Here's how the part is built. I have some questions about the finished solid (model axes, mm). Give positions to 0.01 mm unless a question says otherwise; leave off trailing zeros. Order: outer loops, then holes, each group sorted by start corner. A loop starts at its lowest first (then second) coordinate and runs counter-clockwise, first axis right, second up.
from build123d import *

# Parameters (mm, degrees)
MODEL_R             = 1.587496825
BOSS_EXTRUDE1_DEPTH = 2


with BuildPart() as part:
    # Model → Boss-Extrude1 (new body)
    with BuildSketch(Plane.XY):
        with BuildLine():
            Line((-146.653910016, 921.021419751), (-146.653491939, 987.021287754))
            Line((-146.653491939, 987.021287754), (-147.399894202, 987.021287754))
            ThreePointArc((-147.399894202, 987.021287754), (-150.935437408, 988.485719341), (-152.399999963, 992.021208297))
            ThreePointArc((-152.399999963, 992.021208297), (-153.278698205, 994.142573511), (-155.400063419, 995.021271753))
            Line((-155.400063419, 995.021271753), (-209.399816512, 995.021271753))
            ThreePointArc((-209.399816512, 995.021271753), (-211.521116241, 994.142638994), (-212.399879965, 992.021393514))
            ThreePointArc((-212.399879965, 992.021393514), (-213.864303366, 988.485858493), (-217.399777355, 987.021287754))
            ThreePointArc((-217.399777355, 987.021287754), (-220.228264308, 985.849690097), (-221.399861964, 983.021203145))
            Line((-221.399861964, 983.021203145), (-221.399861964, 925.021411752))
            ThreePointArc((-221.399861964, 925.021411752), (-220.228216634, 922.192969733), (-217.39973512, 921.02141975))
            ThreePointArc((-217.39973512, 921.02141975), (-213.864288435, 919.55683408), (-212.399879966, 916.021313993))
            ThreePointArc((-212.399879966, 916.021313993), (-211.521116244, 913.900068513), (-209.399816515, 913.021435753))
            Line((-209.399816515, 913.021435753), (-155.506885764, 913.021435753))
            ThreePointArc((-155.506885764, 913.021435753), (-155.475395221, 913.097173017), (-155.399490011, 913.128256561))
            ThreePointArc((-155.399490011, 913.128256561), (-155.324999759, 913.097438787), (-155.293258, 913.023337548))
            ThreePointArc((-155.293258, 913.023337548), (-153.267730715, 913.91115848), (-152.400955638, 915.945780743))
            ThreePointArc((-152.400955638, 915.945780743), (-152.427675956, 915.951027262), (-152.450799863, 915.965407327))
            ThreePointArc((-152.450799863, 915.965407327), (-152.470357006, 916.048810735), (-152.399429358, 916.096851124))
            ThreePointArc((-152.399429358, 916.096851124), (-150.946546283, 919.545844687), (-147.506710495, 921.020278673))
            ThreePointArc((-147.506710495, 921.020278673), (-147.476166718, 921.096209628), (-147.400849891, 921.128237863))
            ThreePointArc((-147.400849891, 921.128237863), (-147.324698014, 921.09729172), (-147.293071814, 921.021419751))
            Line((-147.293071814, 921.021419751), (-146.653910016, 921.021419751))
        make_face()
        with Locations((-208.399887964, 918.965401326)):
            Circle(MODEL_R, mode=Mode.SUBTRACT)
        with Locations((-157.399989964, 918.965401326)):
            Circle(MODEL_R, mode=Mode.SUBTRACT)
        with Locations((-208.399887964, 988.965261326)):
            Circle(MODEL_R, mode=Mode.SUBTRACT)
        with Locations((-157.399989964, 988.965261326)):
            Circle(MODEL_R, mode=Mode.SUBTRACT)
    extrude(amount=BOSS_EXTRUDE1_DEPTH)


solid = part.part
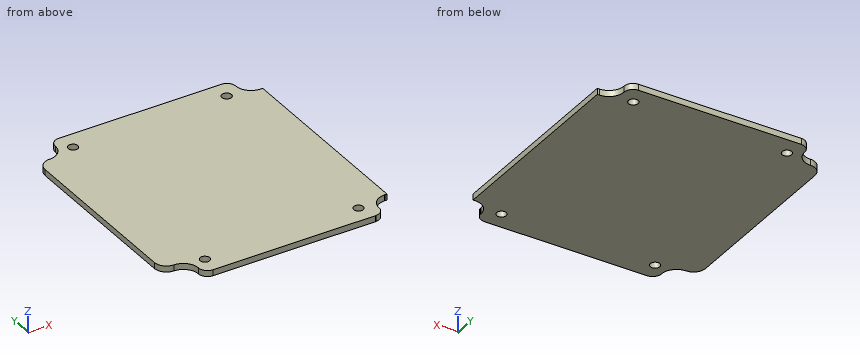
Q1. I'm going to push a flat-ended pin straight in: P1, Ø0.8, axis at x = -147, z = 1, coming from the +Y side. Where does the tip first touch, or does it pass through?
Filled sheet:
P1: stops at y = 987.02
Q2. If we section it at A-A on z = 0.3: Give the number of separate pieces and of enclosed holes in the cut face, plus the area to 3 significant figures.
Filled sheet:
separate pieces: 1
enclosed holes: 4
area: 5,870 mm2
Q3. I need wall thicknesses on L1, parallel to Y at x = -208, z = 1.25; L2, parallel to Y at x = -156, z = 0.2; L3, parallel to Y at x = -152, z = 0.8. Which ranges of each line are inside material? Lowest first, please.
Filled sheet:
L1: y = 913.02 to 917.43, 920.5 to 987.43, 990.5 to 995.02
L2: y = 913.02 to 918.22, 919.71 to 988.22, 989.71 to 995.02
L3: y = 917.98 to 990.06
Q4. If we section it at B-B on x = -151: List the corners of the cut face in (y, z) for me, plus the area to 3 significant figures.
Filled sheet:
outline: (919.49, 0) - (988.55, 0) - (988.55, 2) - (919.49, 2) - close
area: 138 mm2
